Here's how the part is built. I have some questions about the finished solid (model axes, mm). A direction names the side the tool comes from. Coordinates: 2 decimals unless noted, no trailing zeros. Loops run counter-clockwise (first coordinate to the right, second up) from the corner with the lowest first, then second, coordinate; pieces in that order, holes last. Notation, with made-up numbers: (27.25, 56.25) -> (78.25, 56.25) arc R31 ccw to (78.25, 87.25) -> close; hole circle Ø10 at (58, -37.5). An arc over 180 degrees is marked (long way). Use CSV: the item, a comma, the result in double quotes. Start each with the question number.
from build123d import *

# Parameters (mm, degrees)
F0_R     = 12.7
F0_R_2   = 3.175
F1_DEPTH = 1.27
F2_R     = 8.8060698198
F2_R_2   = 3.175
F3_DEPTH = 5.55625
F4_R     = 12.8157676945
F4_R_2   = 8.8060698198
F4_R_3   = 3.175
F5_DEPTH = 1.27


with BuildPart() as f1:
    # F0 (on Top) → F1 (new body)
    with BuildSketch(Plane.XY):
        with Locations((-24.458033964, 35.4546681046)):
            Circle(F0_R)
        with Locations((-24.458033964, 35.4546681046)):
            Circle(F0_R_2, mode=Mode.SUBTRACT)
    extrude(amount=F1_DEPTH)

    # F2 (on face) → F3 (join)
    with BuildSketch(Plane.XY.offset(1.27)):
        with Locations((-24.458033964, 35.4546681046)):
            Circle(F2_R)
        with Locations((-24.458033964, 35.4546681046)):
            Circle(F2_R_2, mode=Mode.SUBTRACT)
    extrude(amount=F3_DEPTH)

    # F4 (on face) → F5 (join)
    with BuildSketch(Plane.XY.offset(6.82625)):
        with Locations((-24.458033964, 35.4546681046)):
            Circle(F4_R)
        with Locations((-24.458033964, 35.4546681046)):
            Circle(F4_R_2, mode=Mode.SUBTRACT)
        with Locations((-24.458033964, 35.4546681046)):
            Circle(F4_R_2)
        with Locations((-24.458033964, 35.4546681046)):
            Circle(F4_R_3, mode=Mode.SUBTRACT)
    extrude(amount=F5_DEPTH)


solid = f1.part
1) Thinking about a two-plate mould opening in Z: for faces 4 (the face through (-22, 33, 8.096)), 5 (the face through (-21.8, 44.2, 6.826)), 6 (the face through (-22, 33, 0)), 7 (the face through (-27.236, 22.944, 7.452)), which applies, pulls with the +Z half, pulls with the -Z half, needs draft (parallel to the pull), parting line crosses it, or undercut?
2) I want a section at C-C, the plane x = -31.5. Please give me the cut outline in (y, z), plus the area to 3 significant figures.
3) For P1, Ø1, axis at x = -23, z = 1.5, coming from the +Y side; P2, Ø3, axis at x = -31.5, z = 3, coming from the -Y side; P3, Ø3, axis at y = 28, z = 2.5, coming from the +X side, each with a flat end and sliding along its axis, tell me the tip position at first contact or that it passes through.
4) Which directions (+Z, -Z, +X, -X, +Y, -Y) give clear straight access to the entire face, cutting with the end or side of a thin tool? Please do faces 1 (the face through (-33.818, 44.038, 0.626)), 2 (the face through (-21.8, 44.1, 1.27)), 3 (the face through (-22.75, 38.13, 3.99)).
5) Please list where these lines run through material, in increasing order: L1, parallel to Z at x = -34, y = 37; L2, parallel to X at y = 35.75, z = 1.5; L3, parallel to X at y = 37.5, z = 3. Write a range as [from, to].
6) I want a section at A-A, the plane x = -26.5. Please give me the cut outline in (y, z).
7) I want a section at B-B, the plane y = 34. Please give me the cut outline in (x, z), plus the area to 3 significant figures.
8) I want a section at D-D, the plane y = 46. Please give me the cut outline in (x, z).
Return value:
1,face 4,"pulls with the +Z half"
1,face 5,"undercut"
1,face 6,"pulls with the -Z half"
1,face 7,"needs draft"
2,outline,"(24.75, 6.83) -> (30.17, 6.83) -> (30.17, 1.27) -> (24.89, 1.27) -> (24.89, 0) -> (46.02, 0) -> (46.02, 1.27) -> (40.74, 1.27) -> (40.74, 6.83) -> (46.16, 6.83) -> (46.16, 8.1) -> (24.75, 8.1) -> close"
2,area,"113 mm²"
3,P1,"stops at y = 48.11"
3,P2,"stops at y = 28.61"
3,P3,"stops at x = -13.61"
4,face 1,"-Z"
4,face 2,"none"
4,face 3,"+Z, -Z"
5,L1,"z = [0, 1.27], [6.83, 8.1]"
5,L2,"x = [-33.26, -27.62], [-21.3, -15.66]"
5,L3,"x = [-33.02, -26.89], [-22.03, -15.89]"
6,outline,"(22.8, 6.83) -> (26.89, 6.83) -> (26.89, 1.27) -> (22.92, 1.27) -> (22.92, 0) -> (33.02, 0) -> (33.02, 8.1) -> (22.8, 8.1) -> close; (37.89, 0) -> (47.99, 0) -> (47.99, 1.27) -> (44.02, 1.27) -> (44.02, 6.83) -> (48.11, 6.83) -> (48.11, 8.1) -> (37.89, 8.1) -> close"
7,outline,"(-37.19, 6.83) -> (-33.14, 6.83) -> (-33.14, 1.27) -> (-37.07, 1.27) -> (-37.07, 0) -> (-27.28, 0) -> (-27.28, 8.1) -> (-37.19, 8.1) -> close; (-21.64, 0) -> (-11.84, 0) -> (-11.84, 1.27) -> (-15.77, 1.27) -> (-15.77, 6.83) -> (-11.73, 6.83) -> (-11.73, 8.1) -> (-21.64, 8.1) -> close"
7,area,"115 mm²"
8,outline,"(-31.74, 6.83) -> (-17.18, 6.83) -> (-17.18, 8.1) -> (-31.74, 8.1) -> close; (-31.54, 0) -> (-17.38, 0) -> (-17.38, 1.27) -> (-31.54, 1.27) -> close"
